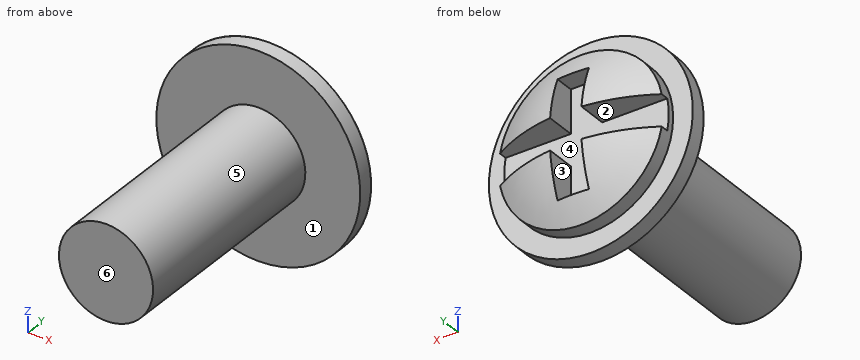
```python
from build123d import *

# Parameters (mm, degrees)
SKETCH_1_R          = 1.5
EXTRUDE_1_DEPTH     = 7
SKETCH_6_R          = 3.25
EXTRUDE_1_2_DEPTH   = 0.5
SKETCH_2_R          = 2.625
EXTRUDE_2_DEPTH     = 1.2
SKETCH_3_W          = 7.004697232
SKETCH_3_H          = 1
CUT_EXTRUDE_1_DEPTH = 1
SKETCH_4_W          = 1
SKETCH_4_H          = 3.75
CUT_EXTRUDE_2_DEPTH = 1


with BuildPart() as part:
    # 草图1 → Extrude 1 (new body)
    with BuildSketch(Plane(origin=(0, 0, 0), x_dir=(1, 0, 0), z_dir=(0, 1, 0))):
        with Locations(Location((0, 0, 0), (0, 0, 270))):
            Circle(SKETCH_1_R)
    extrude(amount=EXTRUDE_1_DEPTH)

    # 草图6 → Extrude 1 2 (add)
    with BuildSketch(Plane(origin=(0, 7, 0), x_dir=(1, 0, 0), z_dir=(0, 1, 0))):
        with Locations(Location((0, 0, 0), (0, 0, 270))):
            Circle(SKETCH_6_R)
    extrude(amount=EXTRUDE_1_2_DEPTH)

    # 草图2 → 拉伸2 (add)
    with BuildSketch(Plane(origin=(0, 7.5, 0), x_dir=(-1, 0, 0), z_dir=(0, 1, 0))):
        with Locations(Location((0, 0, 0), (0, 0, 90))):
            Circle(SKETCH_2_R)
    extrude(amount=EXTRUDE_2_DEPTH)

    # 草图3 → 切除-拉伸1 (cut)
    with BuildSketch(Plane(origin=(0, 8.7, 0), x_dir=(-1, 0, 0), z_dir=(0, 1, 0))):
        Rectangle(SKETCH_3_W, SKETCH_3_H)
    extrude(amount=-CUT_EXTRUDE_1_DEPTH, mode=Mode.SUBTRACT)

    # 草图4 → 切除-拉伸2 (cut)
    with BuildSketch(Plane(origin=(0, 8.7, 0), x_dir=(-1, 0, 0), z_dir=(0, 1, 0))):
        Rectangle(SKETCH_4_W, SKETCH_4_H)
    extrude(amount=-CUT_EXTRUDE_2_DEPTH, mode=Mode.SUBTRACT)

    # 草图5 → 切除-旋转16 (revolve, cut)
    with BuildSketch(Plane(origin=(0, 0, 0), x_dir=(0, 0, -1), z_dir=(1, 0, 0))):
        with BuildLine():
            Line((0, 11.324107024), (-3.685811759, 11.324107024))
            Line((-3.685811759, 11.324107024), (-3.685811759, 7.078578352))
            ThreePointArc((-3.685811759, 7.078578352), (-2.013344014, 8.276728731), (0, 8.7))
            Line((0, 8.7), (0, 11.324107024))
        make_face()
    revolve(axis=Axis((0, -2.105917543, 0), (0, 1, 0)), mode=Mode.SUBTRACT)


solid = part.part
```
Read the model definition and answer for the solid it produces. Units are mm, in the model's axes. Face numbers are marked on the shaded views. A direction names the side the tool comes from. Coordinates: 2 decimals unless noted, no trailing zeros. Order: outer loops, then holes, each group sorted by start corner. A loop starts at its lowest first (then second) coordinate and runs counter-clockwise, first axis right, second up. Notation, with made-up numbers: (87, 7) - (124, 7) arc R17 cw to (124, 32) - close; hole circle Ø7 at (43, -23.5). An arc over 180 degrees is marked (long way). Answer as a JSON object with one key per item and string values. Group by question number.
Item 1: The mould has two halves that part along X. Classify the marked faces 4, 5 and 6: +X half, -X half, draft (parallel to the pull), parting line (faces both ways), or undercut.
Item 2: Section C-C (y = 1) is taken. Give the vertices of the cut face in (x, z), plus the area to 3 significant figures.
Item 3: Consider probe 1 along Y at (x, z) = (0, -1); probe 2 along X at (y, z) = (2.75, 0); probe 3 along Y at (x, z) = (1.75, -2.5). Determine where each line is inside the solid, lowest interval first. Write a range as from..to.
Item 4: A tool of negligible diameter and unlimited length cuts with its end or side. For the marked faces 1, 2 and 3, from which of +Z, -Z, +X, -X, +Y, -Y can it reach the whole face along a straight path? Write none if from no direction.
Item 5: Flat-ended cylindrical pins translate along their axes: P1, Ø3, axis at x = 0, z = 0, coming from the +Y side; P2, Ø0.5, axis at x = 0, y = 8, coming from the -Z side (3 decimals); P3, Ø0.5, axis at x = 1.5, y = 8, coming from the -Z side; P4, Ø0.5, axis at x = 0, y = 8, coming from the +Z side (3 decimals). Find the tip coordinate at first contact, or state that the pin passes through.
Results are:
{
 "1": {"face 4": "undercut", "face 5": "parting line", "face 6": "draft"},
 "2": {"outline": "circle Ø3 at (0, 0)", "area": "7.07 mm^2"},
 "3": {"probe 1": "y = 0..7.7", "probe 2": "x = -1.5..1.5", "probe 3": "y = 7..7.5"},
 "4": {"face 1": "-Y", "face 2": "+X, -X, +Y", "face 3": "+Y"},
 "5": {"P1": "stops at y = 8.65", "P2": "stops at z = -2.625", "P3": "stops at z = -2.31", "P4": "stops at z = 2.625"}
}
